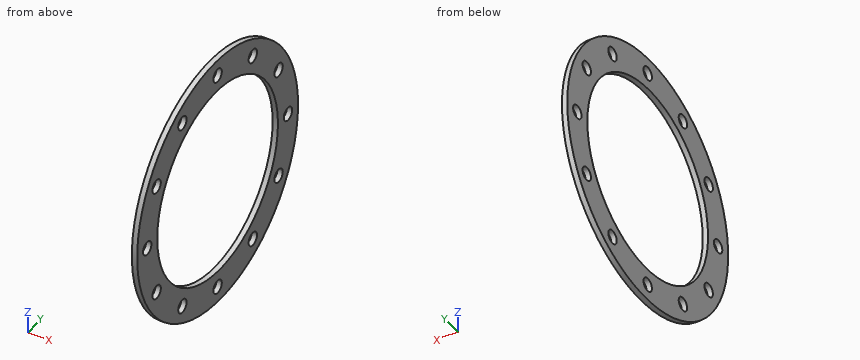
from build123d import *

# Parameters (mm, degrees)
F0_R     = 76.2
F0_R_2   = 3.96875
F0_R_3   = 57.15
F1_DEPTH = 3.175


with BuildPart() as f1:
    # F0 (on Right) → F1 (new body)
    with BuildSketch(Plane.YZ):
        Circle(F0_R)
        with Locations((-33.3375, -57.742244)):
            Circle(F0_R_2, mode=Mode.SUBTRACT)
        with Locations((-57.742244, -33.3375)):
            Circle(F0_R_2, mode=Mode.SUBTRACT)
        with Locations((0, -66.675)):
            Circle(F0_R_2, mode=Mode.SUBTRACT)
        with Locations((33.3375, -57.742244)):
            Circle(F0_R_2, mode=Mode.SUBTRACT)
        with Locations((57.742244, -33.3375)):
            Circle(F0_R_2, mode=Mode.SUBTRACT)
        with Locations((-66.675, 0)):
            Circle(F0_R_2, mode=Mode.SUBTRACT)
        with Locations((-57.742244, 33.3375)):
            Circle(F0_R_2, mode=Mode.SUBTRACT)
        with Locations((-33.3375, 57.742244)):
            Circle(F0_R_2, mode=Mode.SUBTRACT)
        Circle(F0_R_3, mode=Mode.SUBTRACT)
        with Locations((66.675, 0)):
            Circle(F0_R_2, mode=Mode.SUBTRACT)
        with Locations((57.742244, 33.3375)):
            Circle(F0_R_2, mode=Mode.SUBTRACT)
        with Locations((0, 66.675)):
            Circle(F0_R_2, mode=Mode.SUBTRACT)
        with Locations((33.3375, 57.742244)):
            Circle(F0_R_2, mode=Mode.SUBTRACT)
    extrude(amount=F1_DEPTH)


solid = f1.part
The listing builds one solid part. Answer for the finished solid, in the listing's coordinates (mm). Round coordinates to 2 decimals unless told otherwise and drop trailing zeros. Order: outer loops, then holes, each group sorted by start corner. A loop starts at its lowest first (then second) coordinate and runs counter-clockwise, first axis right, second up. Notation, with made-up numbers: (68.25, -24) -> (83.25, -24) arc R27 cw to (83.25, 6) -> close; hole circle Ø9 at (13.5, -9). An arc over 180 degrees is marked (long way). One line per item, written item: value.
Item 1: Find section A-A, the plane z = 0. Give the vertices of the cut face in (x, y) (3 decimals), then the cut area to 3 significant figures.
Taken from the geometry:
outline: (0, -76.2) -> (3.175, -76.2) -> (3.175, -70.644) -> (0, -70.644) -> close; (0, -62.706) -> (3.175, -62.706) -> (3.175, -57.15) -> (0, -57.15) -> close; (0, 57.15) -> (3.175, 57.15) -> (3.175, 62.706) -> (0, 62.706) -> close; (0, 70.644) -> (3.175, 70.644) -> (3.175, 76.2) -> (0, 76.2) -> close
area: 70.6 mm2
Item 2: Given P1, Ø9, axis at y = -33.34, z = -57.74, coming from the +X side (3 decimals); P2, Ø1.5, axis at x = 2, y = 5, coming from the -Z side; P3, Ø1.5, axis at x = 2, y = 6, coming from the -Z side, each flat-ended and moving along its own axis, determine where each tip first touches the part or whether it passes through.
Taken from the geometry:
P1: stops at x = 3.175
P2: stops at z = -76.08
P3: stops at z = -76.02
Item 3: Straight lines are drawn through the part: L1, parallel to Z at x = 1, y = 0; L2, parallel to Y at x = 2.85, z = 59.5; L3, parallel to Z at x = 2.1, y = 32. For each, find the intervals that lie inside material, in ascending order.
Taken from the geometry:
L1: z = -76.2 to -70.64, -62.71 to -57.15, 57.15 to 62.71, 70.64 to 76.2
L2: y = -47.6 to -36.9, -29.78 to 29.78, 36.9 to 47.6
L3: z = -69.16 to -61.48, -54.01 to -47.35, 47.35 to 54.01, 61.48 to 69.16
Item 4: Find section D-D, the plane x = 0.65. State how many separate pieces and enclosed holes the cut face has, then the cut area to 3 significant figures.
Taken from the geometry:
separate pieces: 1
enclosed holes: 13
area: 7,390 mm2
Item 5: Find section C-C, the plane y = 46. Give the vertices of the cut face in (x, z) (3 decimals).
Taken from the geometry:
outline: (0, -60.749) -> (3.175, -60.749) -> (3.175, -33.913) -> (0, -33.913) -> close; (0, 33.913) -> (3.175, 33.913) -> (3.175, 60.749) -> (0, 60.749) -> close
